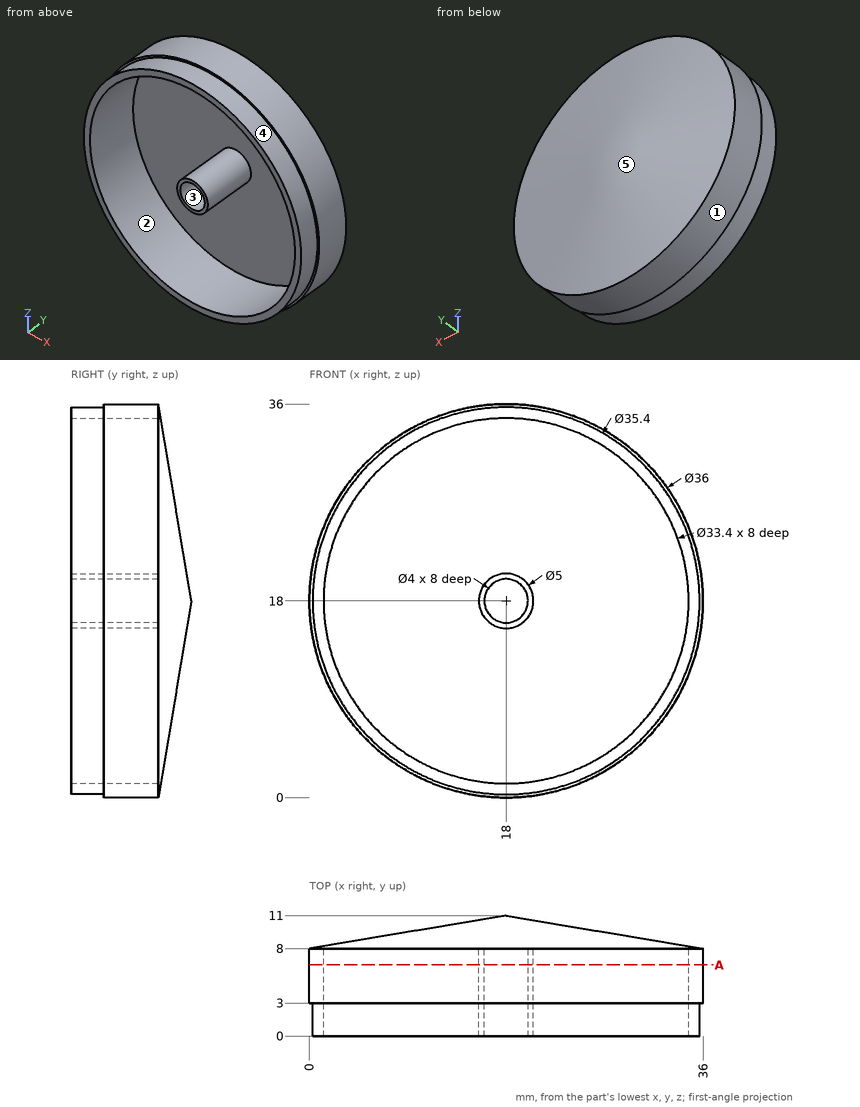
Input: dimensioned drawing with shaded views. Units: mm. Origin: part minimum x, y, z. A direction names the side the tool comes from. Round coordinates to 2 decimals unless told otherwise and drop trailing zeros. Order: outer loops, then holes, each group sorted by start corner. A loop starts at its lowest first (then second) coordinate and runs counter-clockwise, first axis right, second up. Notation, with made-up numbers: (80.25, 37) - (127.25, 37) arc R28 ccw to (127.25, 65) - close; hole circle Ø6 at (-17, 81.25). An arc over 180 degrees is marked (long way). Use CSV: the item, a comma, the result in double quotes. Start each with the question number.
Q1. First-contact query: pin 1 (6 mm diameter, centred on x = 17, z = 25.5, fed in from -Y); pin 2 (1.5 mm diameter, centred on y = 2, z = 24.5, fed in from -X); pin 3 (2 mm diameter, centred on x = 31, z = 15, fed in from +Y). Flat tips, straight axial feed; report the tip coordinate or a pass-through.
Q2. Access query for the marked faces 4 and 5. Directions: +Z, -Z, +X, -X, +Y, -Y. A direction counts if a zero-diameter tool reaches every point of the face in a straight line with its end or side. Return the directions, or none.
Q3. Section query A-A (y = 6.5). Return loops of the section in (x, z), and give its area (3 significant figures).
Q4. Material intervals for line 1 along X through (y, z) = (5, 18); line 2 along X through (y, z) = (2.25, 18); line 3 along Z through (x, y) = (26, 3.75), sorted ascending. Write a range as from..to.
Q5. Mould query, pull axis Z, two halves, no side actions, for the marked faces 1, 2 and 3. Classes: +Z half, -Z half, draft (parallel to the pull), parting line (faces both ways), or undercut.
Result set:
1,pin 1,"stops at y = 8"
1,pin 2,"stops at x = 1.26"
1,pin 3,"stops at y = 8.94"
2,face 4,"-Y"
2,face 5,"+Y"
3,outline,"circle Ø36 at (18, 18); circle Ø5 at (18, 18); hole circle Ø33.4 at (18, 18); hole circle Ø4 at (18, 18)"
3,area,"149 mm2"
4,line 1,"x = 0..1.3, 15.5..16, 20..20.5, 34.7..36"
4,line 2,"x = 0.3..1.3, 15.5..16, 20..20.5, 34.7..35.7"
4,line 3,"z = 1.88..3.34, 32.66..34.12"
5,face 1,"parting line"
5,face 2,"undercut"
5,face 3,"undercut"
